from build123d import *

# Parameters (mm, degrees)
F0_R     = 38.1
F1_DEPTH = 6.35
F2_R     = 3.175
F2_R_2   = 4.7625
F3_DEPTH = 25.4
F4_SIZE  = 1.27


# Not quite as in the source:
# - a length typed as a fraction of an inch, garbled in the dataset ("3 / 203.2 mm" for 3/8 in), is restored


with BuildPart() as f1:
    # F0 (on Top) → F1 (new body)
    with BuildSketch(Plane.XY):
        Circle(F0_R)
    extrude(amount=F1_DEPTH)

    # F2 (on Top) → F3 (cut)
    with BuildSketch(Plane.XY):
        with Locations((-31.7926891148, 0)):
            Circle(F2_R)
        with Locations((31.7926891148, 0)):
            Circle(F2_R)
        Circle(F2_R_2)
    extrude(amount=F3_DEPTH, mode=Mode.SUBTRACT)

    # F4
    f4_edges = [f1.edges().sort_by_distance(p)[0] for p in [
        (-38.1, 0, 0),
    ]]
    chamfer(f4_edges, length=F4_SIZE)


solid = f1.part
Input: part model. Units: mm. Frame: model coordinates. Coordinates: 2 decimals unless noted, no trailing zeros. Write each loop counter-clockwise with the first axis right and the second up, starting at its lowest first coordinate (ties: lowest second). Pieces come first, ordered by that corner, then holes. Notation, with made-up numbers: M 50,65 L 75,65 A14 ccw 75,79 Z; hole C 87,68.5 d3. An arc over 180 degrees is marked long. Answer as a JSON object with one key per item and string values. Group by question number.
(1) Section A-A on y = 0. Output: boundary loops of the cut face in (x, z).
(2) Mould query, pull axis Y, two halves, no side actions, for faces 1 (the face through (28.62, 0.14, 3.13)), 2 (the face through (8, 1, 6.35)), 3 (the face through (-30.235, -23.183, 3.774)). Classes: pulls with the +Y half, pulls with the -Y half, needs draft (parallel to the pull), parting line crosses it, or undercut.
(3) Contact query for flat-ended pins moving along their axis: P1, Ø3, axis at y = 14.5, z = 2.5, coming from the -X side; P2, Ø2, axis at y = 29.5, z = 4.5, coming from the -X side; P3, Ø2, axis at x = -21, z = 5.5, coming from the -Y side. Output: stop coordinate, or through.
(4) Section C-C on z = 3.75. Give the number of separate pieces and of enclosed holes in the cut face, plus the area to 3 significant figures.
(5) Section B-B on x = 0. Output: boundary loops of the cut face in (y, z), plus the area to 3 significant figures.
(6) Ray query, line 1 along X through (y, z) = (-1, 5.5); line 2 along Y through (x, z) = (0, 2.5); line 3 along Y through (x, z) = (33, 1). Return the intervals inside material, ascending. Write a range as [from, to].
Result set:
{
 "1": {"outline": "M -38.1,1.27 L -36.83,0 L -34.97,0 L -34.97,6.35 L -38.1,6.35 Z; M -28.62,0 L -4.76,0 L -4.76,6.35 L -28.62,6.35 Z; M 4.76,0 L 28.62,0 L 28.62,6.35 L 4.76,6.35 Z; M 34.97,0 L 36.83,0 L 38.1,1.27 L 38.1,6.35 L 34.97,6.35 Z"},
 "2": {"face 1": "undercut", "face 2": "needs draft", "face 3": "parting line crosses it"},
 "3": {"P1": "stops at x = -35.81", "P2": "stops at x = -25.29", "P3": "stops at y = -32.43"},
 "4": {"separate pieces": "1", "enclosed holes": "3", "area": "4,430 mm2"},
 "5": {"outline": "M -38.1,1.27 L -36.83,0 L -4.76,0 L -4.76,6.35 L -38.1,6.35 Z; M 4.76,0 L 36.83,0 L 38.1,1.27 L 38.1,6.35 L 4.76,6.35 Z", "area": "422 mm2"},
 "6": {"line 1": "x = [-38.09, -34.81], [-28.78, -4.66], [4.66, 28.78], [34.81, 38.09]", "line 2": "y = [-38.1, -4.76], [4.76, 38.1]", "line 3": "y = [-18.5, -2.94], [2.94, 18.5]"}
}
